from build123d import *

# Parameters (mm, degrees)
F1_DEPTH = 63.5
F2_DEPTH = 25.4


with BuildPart() as f1:
    # F0 (on Front) → F1 (new body)
    with BuildSketch(Plane.XZ):
        with BuildLine():
            Line((0, -1.651), (0, 1.651))
            ThreePointArc((0, 1.651), (-1.651, 0), (0, -1.651))
        make_face()
        with BuildLine():
            ThreePointArc((0, -1.651), (1.1674332957, -1.1674332957), (1.651, 0))
            ThreePointArc((1.651, 0), (1.1674332957, 1.1674332957), (0, 1.651))
            Line((0, 1.651), (0, -1.651))
        make_face()
    extrude(amount=-F1_DEPTH)

    # F2 (add): a face of the model
    f2_faces = [f1.faces().sort_by_distance(p)[0] for p in [
        (0, 0, 0),
    ]]
    extrude(f2_faces, amount=F2_DEPTH)


solid = f1.part
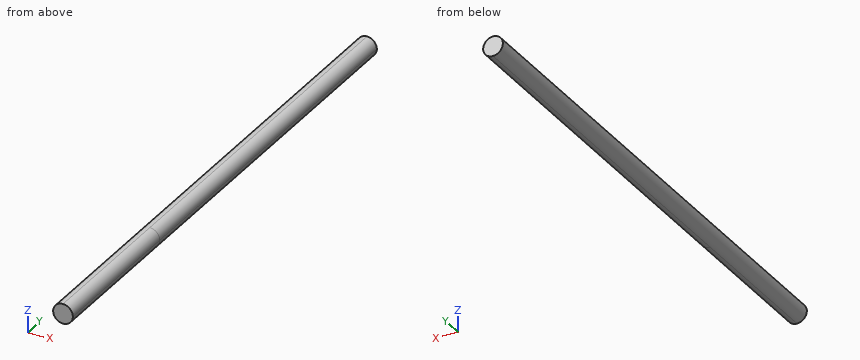
The model under review builds one solid part; all positions refer to its coordinate system, in mm. Round coordinates to 2 decimals unless told otherwise and drop trailing zeros. Write each loop counter-clockwise with the first axis right and the second up, starting at its lowest first coordinate (ties: lowest second). Pieces come first, ordered by that corner, then holes. Notation, with made-up numbers: (61, -16.75) -> (81, -16.75) arc R21 ccw to (81, 13.25) -> close; hole circle Ø7 at (84, -27). An arc over 180 degrees is marked (long way). Answer as a JSON object with one key per item and string values.
1. We need section A-A on y = -10.5. State the section outline as (x, z) points.
Results found:
{"outline": "circle Ø3.3 at (0, 0)"}
2. We need section C-C on z = 1.05. State the section outline as (x, y) points, and give its area (3 significant figures).
Results found:
{"outline": "(-1.27, -25.4) -> (1.27, -25.4) -> (1.27, 63.5) -> (-1.27, 63.5) -> close", "area": "227 mm^2"}
3. We need section B-B on x = -0.5. State the section outline as (y, z) points, and give its area (3 significant figures).
Results found:
{"outline": "(-25.4, -1.57) -> (63.5, -1.57) -> (63.5, 1.57) -> (-25.4, 1.57) -> close", "area": "280 mm^2"}
4. To check wall thickness, follow line 1 along X through (y, z) = (42, 0.15); line 2 along Z through (x, y) = (0.6, 5.5); line 3 along Z through (x, y) = (0.45, -1). State the ranges of each line that lie inside material, in increasing order.
Results found:
{"line 1": "x = -1.64 to 1.64", "line 2": "z = -1.54 to 1.54", "line 3": "z = -1.59 to 1.59"}
